For this review, use the dimensioned drawing (mm, ordinates from the lowest corner) and the shaded views. Coordinates: 2 decimals unless noted, no trailing zeros. Loops run counter-clockwise (first coordinate to the right, second up) from the corner with the lowest first, then second, coordinate; pieces in that order, holes last. Notation, with made-up numbers: M 84.5,-14.5 L 112.5,-14.5 A16 cw 112.5,7.5 Z; hole C -25.5,49 d7. An arc over 180 degrees is marked long. One line per item, written item: value.
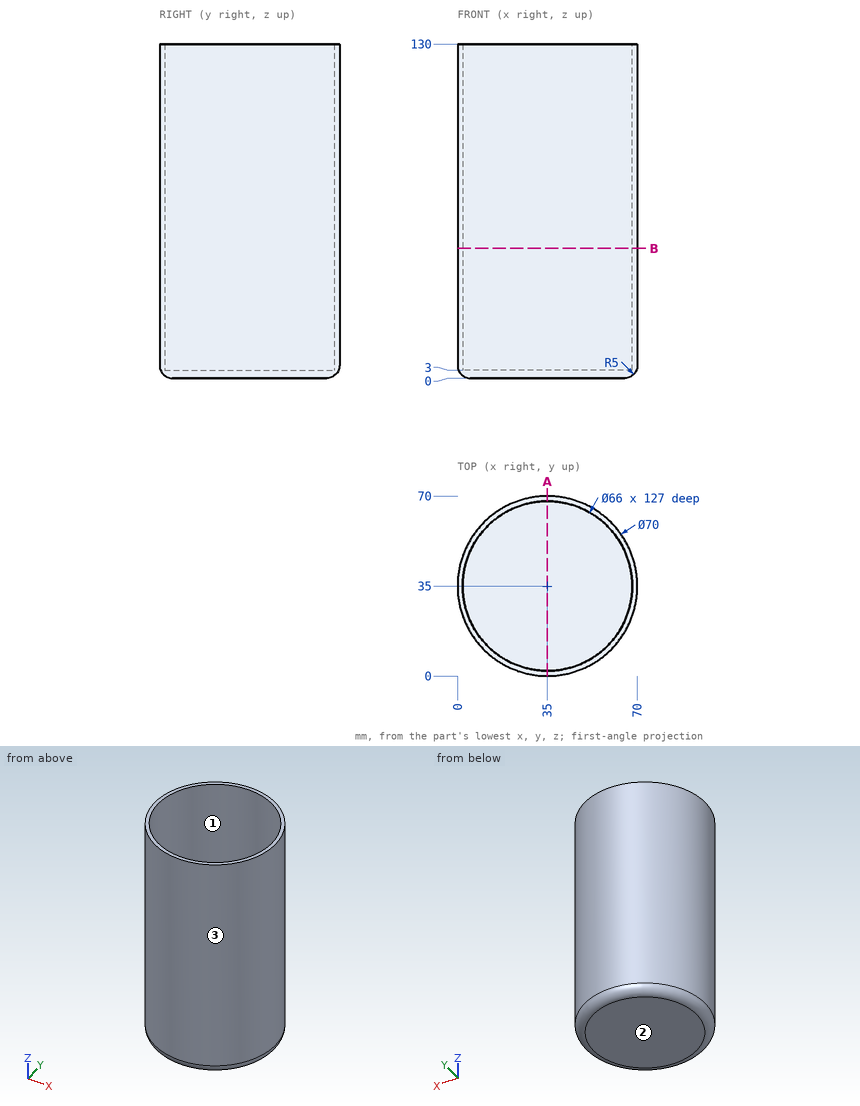
(1) To check wall thickness, follow line 1 along Y through (x, z) = (35, 49.5); line 2 along Z through (x, y) = (19, 24.5); line 3 along Y through (x, z) = (40, 83). State the ranges of each line that lie inside material, in increasing order. Write a range as [from, to].
Reply:
line 1: y = [0, 2], [68, 70]
line 2: z = [0, 3]
line 3: y = [0.36, 2.38], [67.62, 69.64]
(2) We need section B-B on z = 50.5. State the section outline as (x, y) points, then the cut area to 3 significant figures.
Reply:
outline: C 35,35 d70; hole C 35,35 d66
area: 427 mm2
(3) Mouldability with a two-part tool opening along Y and no side actions: class the marked faces 1, 2 and 3 as released by +Y, released by -Y, zero draft, split by the parting line, or undercut.
Reply:
face 1: undercut
face 2: zero draft
face 3: split by the parting line
(4) We need section A-A on x = 35. State the section outline as (y, z) points.
Reply:
outline: M 0,5 A5 ccw 5,0 L 65,0 A5 ccw 70,5 L 70,130 L 68,130 L 68,3 L 2,3 L 2,130 L 0,130 Z
(5) Insertion check: pin 1 (3 mm diameter, centred on x = 57.5, z = 23, fed in from +Y); pin 2 (8 mm diameter, centred on y = 28, z = 78.5, fed in from -X); pin 3 (5 mm diameter, centred on x = 28.5, z = 33, fed in from +Y). Each pin has a flat end and moves straight along its axis. Give the tip position at first contact, or say it passes through.
Reply:
pin 1: stops at y = 63
pin 2: stops at x = 0.13
pin 3: stops at y = 69.77
